```python
from build123d import *

# Parameters (mm, degrees)
SKETCH1_W                  = 12
SKETCH1_H                  = 4
F_6_6_6_6_DIAMETER_HOLE1_D = 6.6
BOSS_EXTRUDE1_DEPTH        = 0.088
FILLET1_R                  = 0.3


with BuildPart() as part:
    # Sketch1 → Revolve1 (revolve)
    with BuildSketch(Plane(origin=(0, 0, 0), x_dir=(-1, 0, 0), z_dir=(0, 0, -1)), mode=Mode.PRIVATE) as revolve1_sk:
        with Locations((-6, 2)):
            Rectangle(SKETCH1_W, SKETCH1_H)
    revolve(revolve1_sk.sketch.rotate(Axis((12, 0, 0), (-1, 0, 0)), 270), axis=Axis((12, 0, 0), (-1, 0, 0)))

    # Ø6.6 (6.6) Diameter Hole1 (through all)
    with Locations(Plane(origin=(12, 0, 0), x_dir=(0, 0, -1), z_dir=(1, 0, 0))):
        with Locations((0, 0)):
            Hole(F_6_6_6_6_DIAMETER_HOLE1_D / 2)

    # Sketch4 → Boss-Extrude1 (add)
    with BuildSketch(Plane(origin=(11.312, 0, 0), x_dir=(0, -1, 0), z_dir=(-1, 0, 0))):
        with BuildLine():
            Line((1.894835085, 0.64), (3.237344591, 0.64))
            ThreePointArc((3.237344591, 0.64), (-3.3, 0), (3.237344591, -0.64))
            Line((3.237344591, -0.64), (1.894835085, -0.64))
            ThreePointArc((1.894835085, -0.64), (2, 0), (1.894835085, 0.64))
        make_face()
    extrude(amount=-BOSS_EXTRUDE1_DEPTH)

    # Sketch5 → Cut-Revolve1 (revolve, cut)
    with BuildSketch(Plane(origin=(0, 0, 0), x_dir=(-1, 0, 0), z_dir=(0, 0, -1)), mode=Mode.PRIVATE) as cut_revolve1_sk:
        Polygon((-11.4, 2), (-11.4, 0), (0, 0), (0, 3.3), (-0.6, 3.3), (-0.6, 2), align=None)
    revolve(cut_revolve1_sk.sketch.rotate(Axis((11.4, 0, 0), (-1, 0, 0)), 90), axis=Axis((11.4, 0, 0), (-1, 0, 0)), mode=Mode.SUBTRACT)

    # Fillet1
    fillet1_edges = [part.edges().sort_by_distance(p)[0] for p in [
        (0, 0, -4),
        (12, 0, -4),
    ]]
    fillet(fillet1_edges, radius=FILLET1_R)


solid = part.part
```
CAD build for the part. Positions are in the model's coordinates, mm. Round coordinates to 2 decimals unless told otherwise and drop trailing zeros. Write each loop counter-clockwise with the first axis right and the second up, starting at its lowest first coordinate (ties: lowest second). Pieces come first, ordered by that corner, then holes. Notation, with made-up numbers: (15.5, -3.75) - (37.5, -3.75) arc R14 ccw to (37.5, 11.25) - close; hole circle Ø1 at (75.25, 70). An arc over 180 degrees is marked (long way). Return JSON: item names as keys, results as strings. Group by question number.
Item 1: Band-saw the part on B-B on z = 0. List the corners of the cut face in (x, y).
Item 2: Mould opens along Y. For faces 1 (the face through (5.92, -3.905, -0.867)), 2 (the face through (5.92, 0.99, 3.15)) say: +Y half, -Y half, draft (parallel to the pull), parting line (faces both ways), or undercut.
Item 3: Flat gauge pins, fed straight in: pin 1 Ø3 at (y, z) = (0, 0) entering from -X; pin 2 Ø3 at (x, y) = (5.5, -3) entering from -Z. Where does each tip first touch, or does it go through?
Item 4: Band-saw the part on A-A on y = 0. List the corners of the cut face in (x, z).
Item 5: Probe probe 1 along Y at (x, z) = (7.75, 0); probe 2 along Y at (x, z) = (1, -2); probe 3 along Z at (x, y) = (3.75, 1.5). List the from-to ranges inside material, lowest first.
Item 6: Band-saw the part on C-C on x = 3. List the corners of the cut face in (y, z).
Resolved:
{
 "1": {"outline": "(0, -3.7) arc R0.3 ccw to (0.3, -4) - (11.7, -4) arc R0.3 ccw to (12, -3.7) - (12, -3.3) - (0, -3.3) - close; (0, 3.3) - (11.31, 3.3) - (11.31, 2) - (11.4, 2) - (11.4, 3.3) - (12, 3.3) - (12, 3.7) arc R0.3 ccw to (11.7, 4) - (0.3, 4) arc R0.3 ccw to (0, 3.7) - close"},
 "2": {"face 1": "parting line", "face 2": "undercut"},
 "3": {"pin 1": "passes through", "pin 2": "stops at z = -3.71"},
 "4": {"outline": "(0, -3.7) arc R0.3 ccw to (0.3, -4) - (11.7, -4) arc R0.3 ccw to (12, -3.7) - (12, -3.3) - (11.4, -3.3) - (11.4, -2) - (11.31, -2) - (11.31, -3.3) - (0, -3.3) - close; (0, 3.3) - (11.31, 3.3) - (11.31, 2) - (11.4, 2) - (11.4, 3.3) - (12, 3.3) - (12, 3.7) arc R0.3 ccw to (11.7, 4) - (0.3, 4) arc R0.3 ccw to (0, 3.7) - close"},
 "5": {"probe 1": "y = -4 to -3.3, 3.3 to 4", "probe 2": "y = -3.46 to -2.62, 2.62 to 3.46", "probe 3": "z = -3.71 to -2.94, 2.94 to 3.71"},
 "6": {"outline": "circle Ø8 at (0, 0); hole circle Ø6.6 at (0, 0)"}
}
